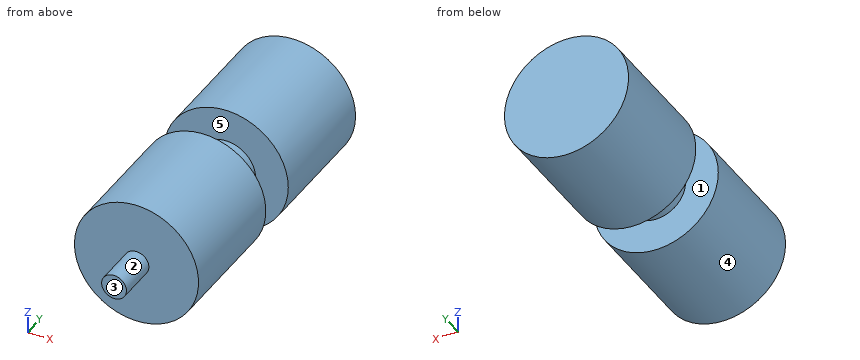
Autodesk Inventor part; units mm, degrees
ref_plane "YZ Plane" through (0, 0, 0) normal (1, 0, 0) x (0, 1, 0)
ref_plane "XZ Plane" through (0, 0, 0) normal (0, 1, 0) x (-1, 0, 0)
ref_plane "XY Plane" through (0, 0, 0) normal (0, 0, 1) x (1, 0, 0)
sketch "スケッチ1" plane through (0, 0, 0) normal (0, 1, 0) x (-1, 0, 0)
  circle A0 centre (0, 0) radius 3
  circle A1 centre (0, 0) radius 15
  dimension "d0" = 6
  dimension "d1" = 30
extrude "押し出し1" add sketch "スケッチ1" along normal blind 30 contours A0 | A1
sketch "スケッチ2" plane through (0, 0, 0) normal (0, -1, 0) x (1, 0, 0)
  circle A0 centre (0, 0) radius 3
  dimension "d4" = 6
extrude "押し出し2" add sketch "スケッチ2" along normal blind 10
sketch "スケッチ3" plane through (0, 30, 0) normal (0, 1, 0) x (1, 0, 0)
  circle A0 centre (0, 0) radius 3
  dimension "d7" = 6
extrude "押し出し3" add sketch "スケッチ3" along normal blind 10
sketch "スケッチ4" plane through (0, 40, 0) normal (0, 1, 0) x (1, 0, 0)
  circle A0 centre (0, 0) radius 15
extrude "押し出し4" add sketch "スケッチ4" along normal blind 30
sketch "スケッチ5" plane through (0, 30, 0) normal (0, 1, 0) x (1, 0, 0)
  circle A0 centre (0, 0) radius 7.0798
extrude "押し出し5" add sketch "スケッチ5" along normal blind 10
Model file for the job. Use its own axes, mm. Face numbers are marked on the shaded views. A direction names the side the tool comes from. Round coordinates to 2 decimals unless told otherwise and drop trailing zeros. Write each loop counter-clockwise with the first axis right and the second up, starting at its lowest first coordinate (ties: lowest second). Pieces come first, ordered by that corner, then holes. Notation, with made-up numbers: M -8.5,85 L 23.5,85 A31 ccw 23.5,123 Z; hole C 89.25,-12.5 d11. An arc over 180 degrees is marked long. Put each result on its own line as item: value.
Item 1: Cut at A-A (x = 13). List the corners of the cut face in (y, z), and give its area (3 significant figures).
Responses:
outline: M 0,-7.48 L 30,-7.48 L 30,7.48 L 0,7.48 Z; M 40,-7.48 L 70,-7.48 L 70,7.48 L 40,7.48 Z
area: 898 mm²
Item 2: Cut at D-D (z = 0). List the corners of the cut face in (x, y), and give its area (3 significant figures).
Responses:
outline: M -15,0 L -3,0 L -3,-10 L 3,-10 L 3,0 L 15,0 L 15,30 L 7.08,30 L 7.08,40 L 15,40 L 15,70 L -15,70 L -15,40 L -7.08,40 L -7.08,30 L -15,30 Z
area: 2,000 mm²
Item 3: Cut at B-B (z = 9.75). List the corners of the cut face in (x, y).
Responses:
outline: M -11.4,0 L 11.4,0 L 11.4,30 L -11.4,30 Z; M -11.4,40 L 11.4,40 L 11.4,70 L -11.4,70 Z
Item 4: Probe L1, parallel to Y at x = 1.5, z = 12; L2, parallel to Y at x = 1, z = 4.75; L3, parallel to Z at x = 0, y = 6.5. List the from-to ranges inside material, lowest first. Write a range as from..to.
Responses:
L1: 0..30, 40..70
L2: 0..70
L3: -15..15
Item 5: Tool access for the marked faces 4 and 5: list every direction of +Z, -Z, +X, -X, +Y, -Y with a clear straight run to the whole face (end or side of a thin tool).
Responses:
face 4: +Y, -Y
face 5: none
Item 6: Mould opens along Y. For the marked faces 1, 2 and 3 say: +Y half, -Y half, draft (parallel to the pull), parting line (faces both ways), or undercut.
Responses:
face 1: undercut
face 2: draft
face 3: -Y half
Item 7: Flat gauge pins, fed straight in: P1, Ø8, axis at y = 53, z = -8, coming from the -X side; P2, Ø2, axis at y = 5.5, z = -2.5, coming from the +X side; P3, Ø6, axis at x = -12, y = 36, coming from the +Z side; P4, Ø12, axis at y = 35, z = -10.5, coming from the -X side. Where does each tip first touch, or does it go through?
Responses:
P1: x = -14.46
P2: x = 14.92
P3: through
P4: x = -13.17
Item 8: Cut at C-C (x = 0). List the corners of the cut face in (y, z), and give its area (3 significant figures).
Responses:
outline: M -10,-3 L 0,-3 L 0,-15 L 30,-15 L 30,-7.08 L 40,-7.08 L 40,-15 L 70,-15 L 70,15 L 40,15 L 40,7.08 L 30,7.08 L 30,15 L 0,15 L 0,3 L -10,3 Z
area: 2,000 mm²
